Design review of the part built by this model. Coordinates are the model's own, in mm. A direction names the side the tool comes from. Give positions to 0.01 mm unless a question says otherwise; leave off trailing zeros. Write each loop counter-clockwise with the first axis right and the second up, starting at its lowest first coordinate (ties: lowest second). Pieces come first, ordered by that corner, then holes.
```python
from build123d import *

# Parameters (mm, degrees)
SKETCH2_R          = 1
CUT_EXTRUDE1_DEPTH = 4
SKETCH3_R          = 1
CUT_EXTRUDE2_DEPTH = 3


with BuildPart() as part:
    # Sketch1 → Revolve1 (revolve)
    with BuildSketch(Plane.XY):
        Polygon((0, 20.601977979), (0, 0), (0, -3.198022021), (1, -3.198022021), (1, -1.398022021), (9.5, -1.398022021), (11.5, 0.601977979), (11.5, 1.601977979), (11, 1.601977979), (11, 2.101977979), (11.5, 2.101977979), (11.5, 3.101977979), (9.5, 3.101977979), (9.5, 3.401977979), (11.5, 3.401977979), (11.5, 13.101977979), (7.5, 17.101977979), (1, 17.101977979), (1, 20.601977979), align=None)
        Polygon((2, 16.101977979), (7.085786438, 16.101977979), (9.423024171, 13.764740246), (9.423024171, 12.764740246), (1, 12.764740246), (1, 15.101977979), (2, 15.101977979), align=None, mode=Mode.SUBTRACT)
    revolve(axis=Axis((0, 20.601977979, 0), (0, -1, 0)))

    # Sketch2 → Cut-Extrude1 (cut)
    with BuildSketch(Plane(origin=(0, 17.101977979, 0), x_dir=(1, 0, 0), z_dir=(0, 1, 0))):
        with Locations((0, -4.5)):
            Circle(SKETCH2_R)
        with Locations((-4.5, 0)):
            Circle(SKETCH2_R)
        with Locations((0, 4.5)):
            Circle(SKETCH2_R)
        with Locations((4.5, 0)):
            Circle(SKETCH2_R)
        with BuildLine():
            Line((-3, 9), (-3, 16.77943101))
            Line((-3, 16.77943101), (3, 16.77943101))
            Line((3, 16.77943101), (3, 9))
            ThreePointArc((3, 9), (0, 6), (-3, 9))
        make_face()
        with BuildLine():
            Line((6.294228634, 7.098076211), (13.031413516, 10.987791717))
            Line((13.031413516, 10.987791717), (16.031413516, 5.791639294))
            Line((16.031413516, 5.791639294), (9.294228634, 1.901923789))
            ThreePointArc((9.294228634, 1.901923789), (5.196152423, 3), (6.294228634, 7.098076211))
        make_face()
        with BuildLine():
            Line((9.294228634, -1.901923789), (16.031413516, -5.791639294))
            Line((16.031413516, -5.791639294), (13.031413516, -10.987791717))
            Line((13.031413516, -10.987791717), (6.294228634, -7.098076211))
            ThreePointArc((6.294228634, -7.098076211), (5.196152423, -3), (9.294228634, -1.901923789))
        make_face()
        with BuildLine():
            Line((3, -9), (3, -16.77943101))
            Line((3, -16.77943101), (-3, -16.77943101))
            Line((-3, -16.77943101), (-3, -9))
            ThreePointArc((-3, -9), (0, -6), (3, -9))
        make_face()
        with BuildLine():
            Line((-6.294228634, -7.098076211), (-13.031413516, -10.987791717))
            Line((-13.031413516, -10.987791717), (-16.031413516, -5.791639294))
            Line((-16.031413516, -5.791639294), (-9.294228634, -1.901923789))
            ThreePointArc((-9.294228634, -1.901923789), (-5.196152423, -3), (-6.294228634, -7.098076211))
        make_face()
        with BuildLine():
            Line((-9.294228634, 1.901923789), (-16.031413516, 5.791639294))
            Line((-16.031413516, 5.791639294), (-13.031413516, 10.987791717))
            Line((-13.031413516, 10.987791717), (-6.294228634, 7.098076211))
            ThreePointArc((-6.294228634, 7.098076211), (-5.196152423, 3), (-9.294228634, 1.901923789))
        make_face()
    extrude(amount=-CUT_EXTRUDE1_DEPTH, mode=Mode.SUBTRACT)

    # Sketch3 → Cut-Extrude2 (cut)
    with BuildSketch(Plane.XZ.offset(1.398022021)):
        with Locations((0, 6)):
            Circle(SKETCH3_R)
        with Locations((0, -6)):
            Circle(SKETCH3_R)
        with Locations((-8, 0)):
            Circle(SKETCH3_R)
        with Locations((8, 0)):
            Circle(SKETCH3_R)
    extrude(amount=-CUT_EXTRUDE2_DEPTH, mode=Mode.SUBTRACT)


solid = part.part
```
(1) Consider section B-B, the plane y = 5. Give the boundary of the cut face in (x, z).
Resolved:
outline: circle Ø23 at (0, 0)
(2) Clearance check with flat-ended pins moving along their axes: P1, Ø5.5, axis at x = -9, z = -6.5, coming from the +Y side; P2, Ø1.2, axis at x = 8, z = 0, coming from the +Y side; P3, Ø8, axis at x = 1, z = -5, coming from the -Y side. State where each tip first meets the part, or that it passes through.
Resolved:
P1: stops at y = 15.09
P2: stops at y = 17.1
P3: stops at y = -1.4
(3) Tool access review of faces 1 (the face through (-0.434, 15.609, -1.952)), 2 (the face through (-5.37, 16.3, -2.73)), 3 (the face through (-0.33, 16.3, -6.02)), 4 (the face through (-8.8, 0.1, -0.6)): name each direction out of +Z, -Z, +X, -X, +Y, -Y from which nothing blocks a thin tool from reaching the whole face with its end or side.
Resolved:
face 1: none
face 2: +Y
face 3: -Z, +Y
face 4: -Y
(4) Consider section A-A, the plane y = 16.75. Give the boundary of the cut face in (x, z).
Resolved:
outline: (-7.71, -1.5) arc R3 cw to (-5.15, -5.92) arc R7.85 ccw to (-2.55, -7.43) arc R3 cw to (2.55, -7.43) arc R7.85 ccw to (5.15, -5.92) arc R3 cw to (7.71, -1.5) arc R7.85 ccw to (7.71, 1.5) arc R3 cw to (5.15, 5.92) arc R7.85 ccw to (2.55, 7.43) arc R3 cw to (-2.55, 7.43) arc R7.85 ccw to (-5.15, 5.92) arc R3 cw to (-7.71, 1.5) arc R7.85 ccw to start; hole circle Ø2 at (-4.5, 0); hole circle Ø2 at (0, -4.5); hole circle Ø2 at (0, 4.5); hole circle Ø2 at (4.5, 0)
(5) Consider section C-C, the plane z = 4.5. Give the number of separate pieces and of enclosed holes in the cut face, then the cut area to 3 significant figures.
Resolved:
separate pieces: 3
enclosed holes: 0
area: 303 mm2
(6) To check wall thickness, follow L1, parallel to Y at x = -7, z = -0.75; L2, parallel to Y at x = 9.25, z = 6.75; L3, parallel to Z at x = 0, y = 0.05. State the ranges of each line that lie inside material, in increasing order.
Resolved:
L1: y = -1.4 to 12.76, 16.1 to 17.1
L2: y = 0.55 to 1.6, 2.1 to 3.1, 3.4 to 13.1
L3: z = -10.95 to -7, -5 to 5, 7 to 10.95
(7) Mouldability with a two-part tool opening along Y and no side actions: class faces 5 (the face through (2, 17.102, 0)), 6 (the face through (-3, 13.7, 9.6)), 7 (the face through (5.066, 13.147, 7.946)) as pulls with the +Y half, pulls with the -Y half, needs draft (parallel to the pull), parting line crosses it, or undercut.
Resolved:
face 5: pulls with the +Y half
face 6: needs draft
face 7: undercut
